```python
from build123d import *

# Parameters (mm, degrees)
F2_R = 0.5


with BuildPart() as f1:
    # F0 (on Right) → F1 (revolve)
    with BuildSketch(Plane.YZ):
        Polygon((-16, 4), (0, 4), (0, 10), (-4, 10), (-4, 5), (-16, 5), align=None)
    revolve(axis=Axis((0, 0, 0), (0, 1, 0)))

    # F2
    f2_edges = [f1.edges().sort_by_distance(p)[0] for p in [
        (0, -16, -4),
        (0, -4, -5),
        (0, -4, -10),
        (0, 0, -10),
    ]]
    fillet(f2_edges, radius=F2_R)


solid = f1.part
```
Can you work these out from the model? Positions are in its coordinate system, mm. Round coordinates to 2 decimals unless told otherwise and drop trailing zeros. Loops run counter-clockwise (first coordinate to the right, second up) from the corner with the lowest first, then second, coordinate; pieces in that order, holes last. Notation, with made-up numbers: M 0.5,-19 L 10.5,-19 A15 ccw 10.5,-1 Z; hole C 45.25,46 d4. An arc over 180 degrees is marked long. Answer as a JSON object with one key per item and string values. Group by question number.
Q1. Will these pins go through, and if not, where does the flat tip stop? pin 1 (2 mm diameter, centred on x = 5, y = -9, fed in from -Z); pin 2 (1.5 mm diameter, centred on x = 2.5, y = -11.5, fed in from -Z); pin 3 (1 mm diameter, centred on y = -9.5, z = 0.5, fed in from -X).
Q2. Imagine slicing it at A-A, the plane z = 0. Please give me the cut outline in (x, y).
Q3. Imagine slicing it at D-D, the plane y = -2. Please give me the cut outline in (x, z).
Q4. Please list where these lines run through material, in increasing order: L1, parallel to X at y = -12.5, z = 0; L2, parallel to Y at x = 1, z = -9; L3, parallel to X at y = -12.5, z = -0.75.
Q5. Imagine slicing it at B-B, the plane x = 0. Please give me the cut outline in (y, z), then the cut area to 3 significant figures.
Q6. We'd pull the mould along X, two halves only. Please class faces 1 (the cylindrical face through (-4.88, -10.33, -1.08)), 2 (the cylindrical face through (-3.905, -7.642, -0.867)), 3 (the flat face through (-4, -4, 4)): +X half, -X half, draft (parallel to the pull), parting line (faces both ways), or undercut.
Q7. Imagine slicing it at C-C, the plane y = -11. Please give me the cut outline in (x, z), then the cut area to 3 significant figures.
Findings:
{
 "1": {"pin 1": "stops at z = -3", "pin 2": "stops at z = -4.68", "pin 3": "stops at x = -5"},
 "2": {"outline": "M -10,-3.5 A0.5 ccw -9.5,-4 L -5.5,-4 A0.5 cw -5,-4.5 L -5,-16 L -4.5,-16 A0.5 ccw -4,-15.5 L -4,0 L -9.5,0 A0.5 ccw -10,-0.5 Z; M 4,-15.5 A0.5 ccw 4.5,-16 L 5,-16 L 5,-4.5 A0.5 cw 5.5,-4 L 9.5,-4 A0.5 ccw 10,-3.5 L 10,-0.5 A0.5 ccw 9.5,0 L 4,0 Z"},
 "3": {"outline": "C 0,0 d20; hole C 0,0 d8"},
 "4": {"L1": "x = -5 to -4, 4 to 5", "L2": "y = -4 to 0", "L3": "x = -4.94 to -3.93, 3.93 to 4.94"},
 "5": {"outline": "M -16,-5 L -4.5,-5 A0.5 cw -4,-5.5 L -4,-9.5 A0.5 ccw -3.5,-10 L -0.5,-10 A0.5 ccw 0,-9.5 L 0,-4 L -15.5,-4 A0.5 ccw -16,-4.5 Z; M -16,4.5 A0.5 ccw -15.5,4 L 0,4 L 0,9.5 A0.5 ccw -0.5,10 L -3.5,10 A0.5 ccw -4,9.5 L -4,5.5 A0.5 cw -4.5,5 L -16,5 Z", "area": "71.8 mm2"},
 "6": {"face 1": "parting line", "face 2": "undercut", "face 3": "draft"},
 "7": {"outline": "C 0,0 d10; hole C 0,0 d8", "area": "28.3 mm2"}
}
